Verification items for the finished model (mm, model axes). Face numbers are marked on the shaded views. A direction names the side the tool comes from. Coordinates: 2 decimals unless noted, no trailing zeros. Write each loop counter-clockwise with the first axis right and the second up, starting at its lowest first coordinate (ties: lowest second). Pieces come first, ordered by that corner, then holes. Notation, with made-up numbers: M -3.5,-9.5 L 29.5,-9.5 A18 ccw 29.5,12.5 Z; hole C 72.5,14.25 d8. An arc over 180 degrees is marked long. One line per item, written item: value.
```python
from build123d import *
from build123d import SkipClean  # not in build123d's __all__

# Parameters (mm, degrees)
F1_DEPTH = 22.352
F4_DEPTH = 60.326
F5_DEPTH = 18.9992
F6_DEPTH = 18.9992
F8_DEPTH = 18.9992


with BuildPart() as f1:
    # F0 (on Top) → F1 (new body)
    with BuildSketch(Plane.XY):
        Polygon((105.8206515543, 17.5817109668), (-110.7397484457, 17.5817109668), (-110.7397484457, -1.4174890332), (-74.0668755353, -1.4174890332), (-74.0668755353, -23.7440890332), (-110.7397484457, -23.7440890332), (-110.7397484457, -42.7432890332), (0, -42.7432890332), (0, -23.7440890332), (25.1433271915, -23.7440890332), (25.1433271915, -42.7432890332), (105.8206515543, -42.7432890332), align=None)
    extrude(amount=F1_DEPTH)

    # F2 (on face) → F4 (cut, through all)
    with BuildSketch(Plane.XZ.offset(42.7432890332)):
        with BuildLine():
            ThreePointArc((-110.7397484457, 11.4130391755), (-97.9889229317, 11.3240532527), (-91.5876839638, 22.352))
            Line((-91.5876839638, 22.352), (-110.7397484457, 22.352))
            Line((-110.7397484457, 22.352), (-110.7397484457, 11.4130391755))
        make_face()
    extrude(amount=-F4_DEPTH, mode=Mode.SUBTRACT)

    # F2 (on face) → F5 (join)
    with BuildSketch(Plane.XZ.offset(42.7432890332)):
        with BuildLine():
            ThreePointArc((-110.7397484457, 1.0841489351), (-91.0484715271, 4.5005608688), (-82.0626839638, 22.352))
            Line((-82.0626839638, 22.352), (-91.5876839638, 22.352))
            ThreePointArc((-91.5876839638, 22.352), (-97.9889229317, 11.3240532527), (-110.7397484457, 11.4130391755))
            Line((-110.7397484457, 11.4130391755), (-110.7397484457, 1.0841489351))
        make_face()
        with BuildLine():
            Line((-91.5876839638, 22.352), (-82.0626839638, 22.352))
            ThreePointArc((-82.0626839638, 22.352), (-117.5268964005, 40.2034391312), (-110.7397484457, 1.0841489351))
            Line((-110.7397484457, 1.0841489351), (-110.7397484457, 11.4130391755))
            ThreePointArc((-110.7397484457, 11.4130391755), (-110.5864449959, 33.3799467473), (-91.5876839638, 22.352))
        make_face()
    with SkipClean():  # cleaning this boolean's faces spoils the solid; the shape is the same uncleaned
        extrude(amount=-F5_DEPTH)

    # F3 (on face) → F6 (join)
    with BuildSketch(Plane(origin=(0, 17.5817109668, 0), x_dir=(-1, 0, 0), z_dir=(0, 1, 0))):
        with BuildLine():
            Line((91.6125912547, 22.352), (82.0875912547, 22.352))
            ThreePointArc((82.0875912547, 22.352), (91.062929817, 4.5083149326), (110.7397484457, 1.0766086889))
            Line((110.7397484457, 1.0766086889), (110.7397484457, 11.3983864208))
            ThreePointArc((110.7397484457, 11.3983864208), (98.0012877573, 11.331226517), (91.6125912547, 22.352))
        make_face()
        with BuildLine():
            ThreePointArc((110.7397484457, 1.0766086889), (122.1562763221, 9.1023385623), (126.5375912547, 22.352))
            ThreePointArc((126.5375912547, 22.352), (104.3125912547, 44.577), (82.0875912547, 22.352))
            Line((82.0875912547, 22.352), (91.6125912547, 22.352))
            ThreePointArc((91.6125912547, 22.352), (104.3125912547, 35.052), (117.0125912547, 22.352))
            ThreePointArc((117.0125912547, 22.352), (115.3333647377, 16.0406965025), (110.7397484457, 11.3983864208))
            Line((110.7397484457, 11.3983864208), (110.7397484457, 1.0766086889))
        make_face()
    extrude(amount=-F6_DEPTH)

    # F7 (on face) → F8 (join)
    with BuildSketch(Plane.XZ.offset(42.7432890332)):
        with BuildLine():
            Line((44.8509039521, 51.7072044313), (27.5659821928, 51.7072044313))
            ThreePointArc((27.5659821928, 51.7072044313), (29.9657018108, 36.7315861898), (25.1433271915, 22.352))
            Line((25.1433271915, 22.352), (49.9309039521, 22.352))
            Line((49.9309039521, 22.352), (49.9309039521, 46.6272044313))
            ThreePointArc((49.9309039521, 46.6272044313), (48.4430064005, 50.2193068797), (44.8509039521, 51.7072044313))
        make_face()
    extrude(amount=-F8_DEPTH)


solid = f1.part
```
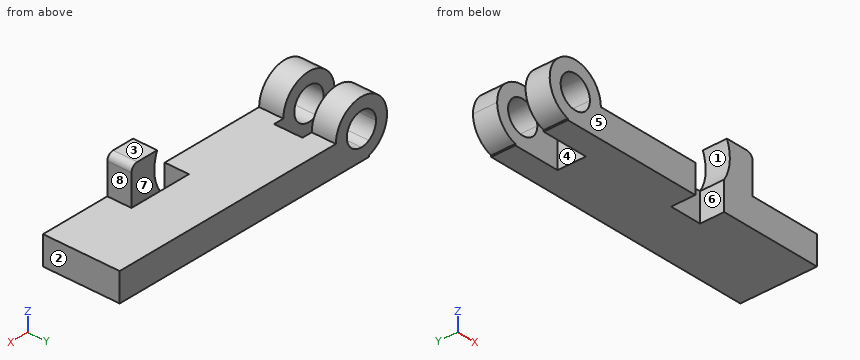
Item 1: Cross-section at B-B, the plane y = 3. Enter the section's corners in (x, z) (3 decimals).
The answers:
outline: M -110.74,0 L 105.821,0 L 105.821,22.352 L -82.088,22.352 A22.225 ccw long -110.74,1.077 Z; hole M -110.74,11.398 L -110.74,11.413 A12.7 ccw -104.3,9.652 A12.7 ccw long Z
Item 2: Access from +Z, -Z, +X, -X, +Y, -Y to the whole of each face (thin tool, end or side, straight path). Record for the marked faces 4, 5, 6, 7 and 8.
The answers:
face 4: +Z, -Z, -X
face 5: +Z, -Z, +X, -X, -Y
face 6: +Z, -Z, -Y
face 7: +Z, +X, -X, +Y
face 8: +Z, +X, +Y, -Y
Item 3: Cross-section at C-C, the plane z = 25. Enter the section's corners in (x, y), and give its area (3 significant figures).
The answers:
outline: M -126.38,-1.42 L -116.73,-1.42 L -116.73,17.58 L -126.38,17.58 Z; M -126.35,-42.74 L -116.71,-42.74 L -116.71,-23.74 L -126.35,-23.74 Z; M -91.89,-1.42 L -82.25,-1.42 L -82.25,17.58 L -91.89,17.58 Z; M -91.87,-42.74 L -82.22,-42.74 L -82.22,-23.74 L -91.87,-23.74 Z; M 26.65,-42.74 L 49.93,-42.74 L 49.93,-23.74 L 26.65,-23.74 Z
area: 1,180 mm²
Item 4: Cross-section at D-D, the plane x = -86.5. Enter the section's corners in (y, z).
The answers:
outline: M -42.74,0 L -23.74,0 L -23.74,35.68 L -42.74,35.68 Z; M -1.42,0 L 17.58,0 L 17.58,35.64 L -1.42,35.64 Z
Item 5: Draft check along X on the marked faces 1, 2 and 3. Enter one of: released by +X, released by -X, zero draft, split by the parting line, or undercut.
The answers:
face 1: undercut
face 2: released by +X
face 3: zero draft
Item 6: Cross-section at A-A, the plane y = -30. Enter the section's corners in (x, z) (3 decimals), and give its area (3 significant figures).
The answers:
outline: M -110.74,0 L 0,0 L 0,22.352 L -82.063,22.352 A22.225 ccw long -110.74,1.084 Z; M 25.143,0 L 105.821,0 L 105.821,22.352 L 49.931,22.352 L 49.931,46.627 A5.08 ccw 44.851,51.707 L 27.566,51.707 A31.743 cw 25.143,22.352 Z; hole C -104.288,22.352 d25.4
area: 5,410 mm²
Item 7: Scan lines: line 1 (X direction, y = -35, z = 13); line 2 (X direction, y = 6.5, z = 22.5); line 3 (X direction, y = -33.5, z = 25). Record each from-to range of solid material in increasing order.
The answers:
line 1: x = -124.45 to -112.88, -95.7 to 0, 25.14 to 105.82
line 2: x = -126.54 to -117.01, -91.61 to -82.09
line 3: x = -126.35 to -116.71, -91.87 to -82.22, 26.65 to 49.93
Item 8: Go/stop test with flat-tipped pins: P1, Ø15, axis at y = -37, z = 40, coming from the +X side; P2, Ø10, axis at x = 28, y = -4, coming from the +Z side; P3, Ø6.5, axis at y = -13.5, z = 10, coming from the -X side. Record where each tip stops, or that it passes through.
The answers:
P1: stops at x = 49.93
P2: stops at z = 22.35
P3: stops at x = -74.07
